Could you check a few things on this model? Use its own coordinates, in mm. A direction names the side the tool comes from. Round coordinates to 2 decimals unless told otherwise and drop trailing zeros. Loops run counter-clockwise (first coordinate to the right, second up) from the corner with the lowest first, then second, coordinate; pieces in that order, holes last. Notation, with made-up numbers: M -22,-11.5 L -3,-11.5 A24 cw -3,23.5 Z; hole C -11.75,71 d11. An arc over 180 degrees is marked long. Answer in a Markdown table with one row per item.
```python
from build123d import *

# Parameters (mm, degrees)
F1_DEPTH  = 13
F2_T      = -1.75
F3_R      = 2.625
F3_R_2    = 1.25
F3_W      = 30
F3_H      = 1.75
F3_W_2    = 8
F3_H_2    = 2
F4_DEPTH  = 11.25
F5_R      = 3
F5_R_2    = 2
F6_DEPTH  = 2
F7_R      = 1.125
F8_DEPTH  = 2
F10_DEPTH = 2
F11_W     = 10
F11_H     = 1.75
F12_DEPTH = 11.25
F13_W     = 10
F13_H     = 1.75
F14_DEPTH = 1.6
F16_DEPTH = 25
F17_W     = 11.5
F17_H     = 31
F18_DEPTH = 1.751
F19_R     = 2.3
F20_DEPTH = 1.751


with BuildPart() as f1:
    # F0 (on Front) → F1 (new body)
    with BuildSketch(Plane.XZ):
        Polygon((0, 36.5), (0, 0), (110, 0), (110, 56.5), (15, 56.5), (15, 36.5), align=None)
    extrude(amount=F1_DEPTH)

    # F2
    f2_openings = [f1.faces().sort_by_distance(p)[0] for p in [
        (57.409129, -13, 27.324387),
    ]]
    offset(amount=F2_T, openings=f2_openings, kind=Kind.INTERSECTION)

    # F3 (on face) → F4 (join, through all)
    with BuildSketch(Plane.XZ.offset(1.75)):
        with Locations((23, 48.5)):
            Circle(F3_R)
        with Locations((23, 48.5)):
            Circle(F3_R_2, mode=Mode.SUBTRACT)
        with Locations((15, 6.7)):
            Circle(F3_R)
        with Locations((15, 6.7)):
            Circle(F3_R_2, mode=Mode.SUBTRACT)
        with Locations((71, 49.5)):
            Circle(F3_R)
        with Locations((71, 49.5)):
            Circle(F3_R_2, mode=Mode.SUBTRACT)
        with Locations((102, 6)):
            Circle(F3_R)
        with Locations((102, 6)):
            Circle(F3_R_2, mode=Mode.SUBTRACT)
        with Locations((93.25, 26.375)):
            Rectangle(F3_W, F3_H)
        with Locations((62, 37.75)):
            Rectangle(F3_W_2, F3_H_2)
    extrude(amount=F4_DEPTH)

    # F5 (on face) → F6 (cut)
    with BuildSketch(Plane.XY.offset(56.5)):
        with Locations((91, -13)):
            Circle(F5_R)
        with Locations((62, -13)):
            Circle(F5_R_2)
    extrude(amount=-F6_DEPTH, mode=Mode.SUBTRACT)

    # F7 (on face) → F8 (cut)
    with BuildSketch(Plane.XY.offset(38.75)):
        with Locations((62, -13)):
            Circle(F7_R)
    extrude(amount=-F8_DEPTH, mode=Mode.SUBTRACT)

    # F9 (on face) → F10 (cut)
    with BuildSketch(Plane.XY.offset(27.25)):
        with BuildLine():
            Line((94.75, -15), (94.75, -11))
            ThreePointArc((94.75, -11), (86.75, -13), (94.75, -15))
        make_face()
    extrude(amount=-F10_DEPTH, mode=Mode.SUBTRACT)

    # F11 (on face) → F12 (join, through all)
    with BuildSketch(Plane.XZ.offset(1.75)):
        with Locations((51.75, 51.375)):
            Rectangle(F11_W, F11_H)
        with Locations((51.75, 29.625)):
            Rectangle(F11_W, F11_H)
    extrude(amount=F12_DEPTH)

    # F13 (on face) → F14 (cut)
    with BuildSketch(Plane.XZ.offset(13)):
        with Locations((51.75, 51.375)):
            Rectangle(F13_W, F13_H)
        with Locations((51.75, 29.625)):
            Rectangle(F13_W, F13_H)
    extrude(amount=-F14_DEPTH, mode=Mode.SUBTRACT)

    # F15 (on face) → F16 (cut)
    with BuildSketch(Plane.XY.offset(52.25)):
        with BuildLine():
            Line((54.094339151, -11.4), (54.1245706409, -10.3060785062))
            ThreePointArc((54.1245706409, -10.3060785062), (52.9989978467, -9.1500004463), (51.8754865135, -10.3080819977))
            Line((51.8754865135, -10.3080819977), (51.9076095865, -11.4))
            Line((51.9076095865, -11.4), (54.094339151, -11.4))
        make_face()
    extrude(amount=-F16_DEPTH, mode=Mode.SUBTRACT)

    # F17 (on face) → F18 (cut, through all)
    with BuildSketch(Plane.XZ.offset(1.75)):
        with Locations((91, 37.25)):
            Rectangle(F17_W, F17_H)
    extrude(amount=-F18_DEPTH, mode=Mode.SUBTRACT)

    # F19 (on face) → F20 (cut, through all)
    with BuildSketch(Plane.XZ.offset(1.75)):
        with Locations((6.75, 12.9)):
            Circle(F19_R)
        with Locations((55.05, 12.9)):
            Circle(F19_R)
        with Locations((102.95, 12.9)):
            Circle(F19_R)
    extrude(amount=-F20_DEPTH, mode=Mode.SUBTRACT)


solid = f1.part
```
1) I want a section at C-C, the plane x = 102. Please give me the cut outline in (y, z) (3 decimals).
Computed:
| item | result |
|---|---|
| outline | M -13,0 L 0,0 L 0,10.805 L -1.75,10.805 L -1.75,8.625 L -13,8.625 L -13,7.25 L -1.75,7.25 L -1.75,4.75 L -13,4.75 L -13,3.375 L -1.75,3.375 L -1.75,1.75 L -13,1.75 Z; M -13,25.5 L -1.75,25.5 L -1.75,14.995 L 0,14.995 L 0,56.5 L -13,56.5 L -13,54.75 L -1.75,54.75 L -1.75,27.25 L -13,27.25 Z |
2) I want a section at D-D, the plane x = 30.5. Please give me the cut outline in (y, z).
Computed:
| item | result |
|---|---|
| outline | M -13,0 L 0,0 L 0,56.5 L -13,56.5 L -13,54.75 L -1.75,54.75 L -1.75,1.75 L -13,1.75 Z |
3) Will these pins go through, and if not, where does the flat tip stop? P1, Ø4, axis at x = 35, z = 31.5, coming from the -Y side; P2, Ø1.9, axis at y = -8.5, z = 51.5, coming from the -X side; P3, Ø0.9, axis at x = 92, z = 26, coming from the +Y side.
Computed:
| item | result |
|---|---|
| P1 | stops at y = -1.75 |
| P2 | stops at x = 15 |
| P3 | stops at y = -1.75 |
4) I want a section at A-A, the plane x = 62. Please give me the cut outline in (y, z) (3 decimals).
Computed:
| item | result |
|---|---|
| outline | M -13,0 L 0,0 L 0,56.5 L -11,56.5 L -11,54.75 L -1.75,54.75 L -1.75,38.75 L -11.875,38.75 L -11.875,36.75 L -1.75,36.75 L -1.75,1.75 L -13,1.75 Z |
5) If we mould it in two halves opening along Z, with no side actions, what happens to faces 5 (the face through (59, -13, 38)), 6 (the face through (23, -1.75, 49))? For each: released by +Z, released by -Z, zero draft, split by the parting line, or undercut.
Computed:
| item | result |
|---|---|
| face 5 | zero draft |
| face 6 | undercut |
6) I need wall thicknesses on line 1 (Z direction, x = 71, y = -9.5) (3 decimals); line 2 (Z direction, x = 65, y = -2.75); line 3 (Z direction, x = 47.5, y = -2). Which ranges of each line are inside material? Lowest first, please.
Computed:
| item | result |
|---|---|
| line 1 | z = 0 to 1.75, 46.875 to 48.25, 50.75 to 52.125, 54.75 to 56.5 |
| line 2 | z = 0 to 1.75, 36.75 to 38.75, 54.75 to 56.5 |
| line 3 | z = 0 to 1.75, 28.75 to 30.5, 50.5 to 52.25, 54.75 to 56.5 |
7) I want a section at B-B, the plane x = 91. Please give me the cut outline in (y, z).
Computed:
| item | result |
|---|---|
| outline | M -13,0 L 0,0 L 0,21.75 L -1.75,21.75 L -1.75,1.75 L -13,1.75 Z; M -10,54.75 L -1.75,54.75 L -1.75,52.75 L 0,52.75 L 0,56.5 L -10,56.5 Z; M -8.75,25.5 L -1.75,25.5 L -1.75,27.25 L -8.75,27.25 Z |
8) Which directions (+Z, -Z, +X, -X, +Y, -Y) give clear straight access to the entire face, cutting with the end or side of a thin tool? Please do faces 1 (the face through (15, -6, 47)), 2 (the face through (54, 0, 29)), 3 (the face through (62.025, -11.875, 37.764)), 4 (the face through (62, -7, 36.75)).
Computed:
| item | result |
|---|---|
| face 1 | +Z, -X, +Y, -Y |
| face 2 | +Z, -Z, +X, -X, +Y |
| face 3 | +Z, -Y |
| face 4 | -Y |
